The listing builds one solid part. Answer for the finished solid, in the listing's coordinates (mm). Coordinates: 2 decimals unless noted, no trailing zeros. Loops run counter-clockwise (first coordinate to the right, second up) from the corner with the lowest first, then second, coordinate; pieces in that order, holes last. Notation, with made-up numbers: (54, 57.25) - (107, 57.25) arc R8 cw to (107, 68.25) - close; hole circle Ø8 at (32.25, 58.5). An arc over 180 degrees is marked (long way). Return JSON: item names as keys, results as strings. Group by question number.
1. Section B-B (x = 21.5) is taken. Write down the section's boundary in (y, z), and give its area (3 significant figures).
2. Each of these flat-tipped pins is pushed along its axis until it touches: P1, Ø1.6, axis at y = 25, z = 39, coming from the -X side; P2, Ø2, axis at y = -25, z = 29, coming from the +X side; P3, Ø2, axis at x = 25, z = 58, coming from the -Y side. Where does it stop, or does it pass through?
3. Find the intervals of material crossed by line 1 along Y through (x, z) = (-24.5, 54); line 2 along Y through (x, z) = (-20.5, 45.5); line 3 along X through (y, z) = (-21, 71), in increasing order.
4. Section C-C (y = -23) is taken. Write down the section's boundary in (x, z).
5. Section A-A (z = 26) is taken. Write down the section's boundary in (x, y), and give its area (3 significant figures).
```python
from build123d import *

# Parameters (mm, degrees)
SKETCH1_W           = 56
SKETCH1_H           = 56
BOSS_EXTRUDE1_DEPTH = 89
SKETCH2_W           = 9
SKETCH2_H           = 9
CUT_EXTRUDE1_DEPTH  = 89
CIRPATTERN1_COUNT   = 4
FILLET1_R           = 5
FILLET2_R           = 2


with BuildPart() as part:
    # Sketch1 → Boss-Extrude1 (new body)
    with BuildSketch(Plane.XY):
        Rectangle(SKETCH1_W, SKETCH1_H)
    extrude(amount=BOSS_EXTRUDE1_DEPTH)

    # Sketch2 → Cut-Extrude1 (cut)
    with BuildSketch(Plane.XY.offset(89)):
        with Locations((23.5, 23.5)):
            Rectangle(SKETCH2_W, SKETCH2_H)
    cut_extrude1 = extrude(amount=-CUT_EXTRUDE1_DEPTH, mode=Mode.SUBTRACT)

    # CirPattern1: Cut-Extrude1 ×4 about axis
    cirpattern1_axis = Axis((0, 0, 0), (0, 0, 1))
    for i in range(1, CIRPATTERN1_COUNT):
        add(cut_extrude1.rotate(cirpattern1_axis, i * 360 / CIRPATTERN1_COUNT), mode=Mode.SUBTRACT)

    # Fillet1
    fillet1_edges = [part.edges().sort_by_distance(p)[0] for p in [
        (19, 19, 44.5),
        (-19, 19, 44.5),
        (-19, -19, 44.5),
        (19, -19, 44.5),
    ]]
    fillet(fillet1_edges, radius=FILLET1_R)

    # Fillet2
    fillet2_edges = [part.edges().sort_by_distance(p)[0] for p in [
        (19, 28, 44.5),
        (28, 19, 44.5),
        (-28, 19, 44.5),
        (-19, 28, 44.5),
        (-19, -28, 44.5),
        (-28, -19, 44.5),
        (28, -19, 44.5),
        (19, -28, 44.5),
    ]]
    fillet(fillet2_edges, radius=FILLET2_R)


solid = part.part
```
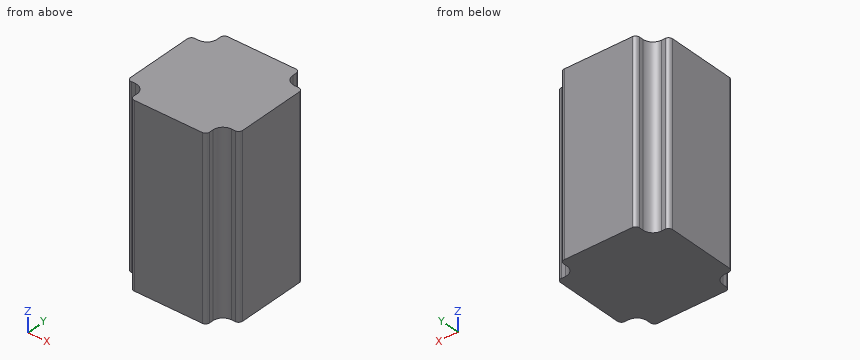
The answers:
{
 "1": {"outline": "(-19.67, 0) - (19.67, 0) - (19.67, 89) - (-19.67, 89) - close", "area": "3,500 mm2"},
 "2": {"P1": "stops at x = -19", "P2": "stops at x = 19", "P3": "stops at y = -19"},
 "3": {"line 1": "y = -19 to 19", "line 2": "y = -20.43 to 20.43", "line 3": "x = -20 to 20"},
 "4": {"outline": "(-19.1, 0) - (19.1, 0) - (19.1, 89) - (-19.1, 89) - close"},
 "5": {"outline": "(-28, -17) arc R2 ccw to (-26, -19) - (-24, -19) arc R5 cw to (-19, -24) - (-19, -26) arc R2 ccw to (-17, -28) - (17, -28) arc R2 ccw to (19, -26) - (19, -24) arc R5 cw to (24, -19) - (26, -19) arc R2 ccw to (28, -17) - (28, 17) arc R2 ccw to (26, 19) - (24, 19) arc R5 cw to (19, 24) - (19, 26) arc R2 ccw to (17, 28) - (-17, 28) arc R2 ccw to (-19, 26) - (-19, 24) arc R5 cw to (-24, 19) - (-26, 19) arc R2 ccw to (-28, 17) - close", "area": "2,830 mm2"}
}
